from build123d import *

# Parameters (mm, degrees)
SKETCH2_W               = 5.4864
SKETCH2_H               = 1.0668
SLOT_DEPTH              = 1.5494
CROQUIS1_R              = 3.23116627
CORTAR_EXTRUIR1_DEPTH   = 12.709724159
CROQUIS4_R              = 1.8034
SALIENTE_EXTRUIR1_DEPTH = 9.525


with BuildPart() as part:
    # BodySke → BaseBody (revolve)
    with BuildSketch(Plane.XY, mode=Mode.PRIVATE) as basebody_sk:
        with BuildLine():
            Line((14.351, 0), (14.351, 1.4605))
            Line((14.351, 1.4605), (13.0683, 2.7432))
            Line((13.0683, 2.7432), (0.735038225, 2.7432))
            ThreePointArc((0.735038225, 2.7432), (0.186944547, 1.419984809), (0, 0))
            Line((0, 0), (14.351, 0))
        make_face()
    revolve(basebody_sk.sketch.rotate(Axis((-12.7, 0, 0), (1, 0, 0)), 90), axis=Axis((-12.7, 0, 0), (1, 0, 0)))

    # Sketch2 → Slot (cut)
    with BuildSketch(Plane(origin=(0, 0, 0), x_dir=(0, 0, -1), z_dir=(1, 0, 0))):
        Rectangle(SKETCH2_W, SKETCH2_H)
    extrude(amount=SLOT_DEPTH, mode=Mode.SUBTRACT)

    # Croquis1 → Cortar-Extruir1 (cut, through all)
    with BuildSketch(Plane.ZY.offset(-11.0744)):
        Circle(CROQUIS1_R)
    extrude(amount=-CORTAR_EXTRUIR1_DEPTH, mode=Mode.SUBTRACT)

    # Croquis4 → Saliente-Extruir1 (add)
    with BuildSketch(Plane(origin=(11.0744, 0, 0), x_dir=(0, 0, -1), z_dir=(1, 0, 0))):
        with Locations(Location((0, 0, 0), (0, 0, 180))):
            Circle(CROQUIS4_R)
    extrude(amount=SALIENTE_EXTRUIR1_DEPTH)


solid = part.part
Geometry: final body of the model. Coordinates: model frame, mm. A direction names the side the tool comes from. Give positions to 0.01 mm unless a question says otherwise; leave off trailing zeros. Write each loop counter-clockwise with the first axis right and the second up, starting at its lowest first coordinate (ties: lowest second). Pieces come first, ordered by that corner, then holes. Notation, with made-up numbers: (11.25, 89.25) -> (47.25, 89.25) arc R11 cw to (47.25, 102.25) -> close; hole circle Ø2 at (-17.75, 23). An arc over 180 degrees is marked (long way). Answer as a JSON object with one key per item and string values.
1. Contact query for flat-ended pins moving along their axis: pin 1 (2 mm diameter, centred on x = 13.5, y = -2, fed in from -Z); pin 2 (1.5 mm diameter, centred on x = 11, y = 1, fed in from -Z); pin 3 (1.2 mm diameter, centred on x = 0.5, z = -1, fed in from +Y). Output: stop coordinate, or through.
Ans:
{"pin 1": "stops at z = -1.5", "pin 2": "stops at z = -2.73", "pin 3": "stops at y = 2.71"}
2. Cut plane D-D on z = -1.3. Output: boundary loops of the cut face in (x, y).
Ans:
{"outline": "(0.18, -0.53) arc R5.33 ccw to (0.74, -2.42) -> (11.07, -2.42) -> (11.07, -1.25) -> (20.6, -1.25) -> (20.6, 1.25) -> (11.07, 1.25) -> (11.07, 2.42) -> (0.74, 2.42) arc R5.33 ccw to (0.18, 0.53) -> (1.55, 0.53) -> (1.55, -0.53) -> close"}
3. Cut plane B-B on z = 0. Output: boundary loops of the cut face in (x, y), and give its area (3 significant figures).
Ans:
{"outline": "(0.03, -0.53) arc R5.49 ccw to (0.74, -2.74) -> (11.07, -2.74) -> (11.07, -1.8) -> (20.6, -1.8) -> (20.6, 1.8) -> (11.07, 1.8) -> (11.07, 2.74) -> (0.74, 2.74) arc R5.49 ccw to (0.03, 0.53) -> (1.55, 0.53) -> (1.55, -0.53) -> close", "area": "92.2 mm^2"}
4. Mould query, pull axis Y, two halves, no side actions, for faces 4 (the flat face through (11.074, -1, 2)), 5 (the cylindrical face through (5.832, -0.824, 2.617)), 6 (the flat face through (1, 0.533, 0)). Classes: pulls with the +Y half, pulls with the -Y half, needs draft (parallel to the pull), parting line crosses it, or undercut.
Ans:
{"face 4": "needs draft", "face 5": "parting line crosses it", "face 6": "undercut"}
5. Cut plane C-C on x = 5.5. Output: boundary loops of the cut face in (y, z), and give its area (3 significant figures).
Ans:
{"outline": "circle Ø5.49 at (0, 0)", "area": "23.6 mm^2"}
6. Ray query, probe 1 along Y at (x, z) = (1, -1.4); probe 2 along X at (y, z) = (-2.1, 0.5); probe 3 along Y at (x, z) = (1.5, -0.7). Return the intervals inside material, ascending. Write a range as from..to.
Ans:
{"probe 1": "y = -2.36..-0.53, 0.53..2.36", "probe 2": "x = 0.44..11.07", "probe 3": "y = -2.65..-0.53, 0.53..2.65"}
7. Cut plane A-A on y = 0. Output: boundary loops of the cut face in (x, z), and give its area (3 significant figures).
Ans:
{"outline": "(1.55, -2.74) -> (11.07, -2.74) -> (11.07, -1.8) -> (20.6, -1.8) -> (20.6, 1.8) -> (11.07, 1.8) -> (11.07, 2.74) -> (1.55, 2.74) -> close", "area": "86.6 mm^2"}
8. Access query for faces 1 (the flat face through (1.549, 0, 0)), 2 (the flat face through (20.599, 0, 0)), 3 (the cylindrical face through (15.77, 1.6, 0.83)). Directions: +Z, -Z, +X, -X, +Y, -Y. A direction counts if a zero-diameter tool reaches every point of the face in a straight line with its end or side. Return the directions, or none.
Ans:
{"face 1": "+Z, -Z, -X", "face 2": "+Z, -Z, +X, +Y, -Y", "face 3": "+X"}
